```python
from build123d import *

# Parameters (mm, degrees)
PAD_DEPTH = 2.5
FILLET_R  = 1


with BuildPart() as part:
    # Sketch → Pad (new body, symmetric)
    with BuildSketch(Plane.YZ):
        with BuildLine():
            ThreePointArc((12.993845, -0.4), (0, 13), (-12.993845, -0.4))
            Line((-12.993845, -0.4), (-9.402299, -1.362352))
            Line((-9.402299, -1.362352), (-9.402299, -4.6))
            Line((-9.402299, -4.6), (-17.402299, -4.6))
            ThreePointArc((17.402299, -4.6), (0, 18), (-17.402299, -4.6))
            Line((17.402299, -4.6), (9.402299, -4.6))
            Line((9.402299, -4.6), (9.402299, -1.362352))
            Line((9.402299, -1.362352), (12.993845, -0.4))
        make_face()
    extrude(amount=PAD_DEPTH, both=True)

    # Fillet
    fillet_edges = [part.edges().sort_by_distance(p)[0] for p in [
        (0, -9.402299, -1.362352),
        (-2.5, -9.402299, -2.981176),
        (-2.5, 0, 13),
        (-2.5, 0, 18),
        (-2.5, 11.198072, -0.881176),
        (-2.5, 9.402299, -2.981176),
        (-2.5, -11.198072, -0.881176),
        (-2.5, -13.402299, -4.6),
        (-2.5, 13.402299, -4.6),
        (2.5, 0, 18),
        (0, 17.402299, -4.6),
        (0, -9.402299, -4.6),
        (2.5, -9.402299, -2.981176),
        (2.5, 0, 13),
        (0, -12.993845, -0.4),
        (0, 12.993845, -0.4),
        (0, 9.402299, -1.362352),
        (0, 9.402299, -4.6),
        (2.5, 9.402299, -2.981176),
        (2.5, 11.198072, -0.881176),
        (2.5, -11.198072, -0.881176),
        (2.5, -13.402299, -4.6),
        (2.5, 13.402299, -4.6),
        (0, -17.402299, -4.6),
    ]]
    fillet(fillet_edges, radius=FILLET_R)


solid = part.part
```
Build history of the part. All positions in model axes, mm. A direction names the side the tool comes from. Give positions to 0.01 mm unless a question says otherwise; leave off trailing zeros. Loops run counter-clockwise (first coordinate to the right, second up) from the corner with the lowest first, then second, coordinate; pieces in that order, holes last.
Item 1: Flat gauge pins, fed straight in: pin 1 (3 mm diameter, centred on y = -13, z = 13.5, fed in from -X); pin 2 (1.2 mm diameter, centred on x = 0.5, z = -2.5, fed in from -Y); pin 3 (1.6 mm diameter, centred on x = 0.5, z = -2.5, fed in from +Y). Where does each tip first touch, or does it go through?
Answers follow:
pin 1: stops at x = -2.47
pin 2: stops at y = -17.9
pin 3: stops at y = 17.92
Item 2: Slice it at B-B, the plane y = 0. List the corners of the cut face in (x, z).
Answers follow:
outline: (-2.5, 14) arc R1 ccw to (-1.5, 13) - (1.5, 13) arc R1 ccw to (2.5, 14) - (2.5, 17) arc R1 ccw to (1.5, 18) - (-1.5, 18) arc R1 ccw to (-2.5, 17) - close
Item 3: Which spindle directions (+Z, -Z, +X, -X, +Y, -Y) get a long thin tool onto all of the face, cutting with end or side? Do faces 4 (the face through (-0.02, -9.7, -4.31)), 5 (the face through (0.021, 12.803, -0.222)), 6 (the face through (2.21, 9.7, -2.85)), 7 (the face through (2.215, 11.291, -1.168)), 8 (the face through (-2.2, 9.69, -2.85)). Say none if no direction does.
Answers follow:
face 4: -Z, +X, -X
face 5: +X, -X
face 6: -Z, +X
face 7: +X
face 8: -Z, -X
Item 4: Drill centre lines: line 1 (Y direction, x = -1.6, z = 4.75); line 2 (Y direction, x = -0.3, z = 10.75); line 3 (Z direction, x = 1.8, y = 3.5). Where is each one in solid material? Low to high.
Answers follow:
line 1: y = -17.36 to -12.11, 12.11 to 17.36
line 2: y = -14.44 to -7.31, 7.31 to 14.44
line 3: z = 12.57 to 17.61
Item 5: Pull direction Y, two halves, no side cores. Call faces 1 (the face through (-0.02, -17.25, -4.37)), 2 (the face through (-2.199, -13.552, -4.315)), 3 (the face through (-2.215, 11.291, -1.168)): released by +Y, released by -Y, zero draft, split by the parting line, or undercut.
Answers follow:
face 1: released by -Y
face 2: zero draft
face 3: undercut
